The model under review builds one solid part; all positions refer to its coordinate system, in mm. A direction names the side the tool comes from. Round coordinates to 2 decimals unless told otherwise and drop trailing zeros. Order: outer loops, then holes, each group sorted by start corner. A loop starts at its lowest first (then second) coordinate and runs counter-clockwise, first axis right, second up. Notation, with made-up numbers: M 49.5,63 L 94.5,63 A27 cw 94.5,85 Z; hole C 71.25,-18 d3. An arc over 180 degrees is marked long. Answer as a JSON object with one key per item and string values. Group by question number.
1. Add section A-A on z = -5.5. State the section outline as (x, y) points.
2. To check wall thickness, follow probe 1 along Z at (x, y) = (-7, 4.5); probe 2 along Z at (x, y) = (5.5, 2); probe 3 along Y at (x, z) = (-18.5, -4). State the ranges of each line that lie inside material, in increasing order. Write a range as [from, to].
3. Add section B-B on y = 6.5. State the section outline as (x, z) points, and give its area (3 significant figures).
4. Add section D-D on z = -2. State the section outline as (x, y) points.
5. Add section C-C on x = 9. State the section outline as (y, z) points, and give its area (3 significant figures).
6. Machinability: for faces 4 (the face through (0.2, 7, -13.2)), 5 (the face through (-24, 5, 12)), 6 (the face through (0, 3, -14)), 7 (the face through (-25.507, 4.65, 3.736)), 8 (the face through (-22.855, 1.15, -11.43)), which of the approach directions +Z, -Z, +X, -X, +Y, -Y give a long, thin tool a straight path to every point of the face, cutting with its end or side? Answer none if there is none.
7. Mouldability with a two-part tool opening along X and no side actions: class faces 1 (the face through (0, 5, -13)), 2 (the face through (23.5, 3, 12)), 3 (the face through (0, 0, 0)) as released by +X, released by -X, zero draft, split by the parting line, or undercut.
8. Clearance check with flat-ended pins moving along their axes: P1, Ø5, axis at x = -6.5, z = 4, coming from the +Y side; P2, Ø1.6, axis at x = -22.5, z = -12, coming from the +Y side; P3, Ø0.6, axis at x = -25, y = 6.5, coming from the -Z side. State where each tip first meets the part, or that it passes through.
```python
from build123d import *

# Parameters (mm, degrees)
SKETCH_1_W          = 52
SKETCH_1_H          = 28
EXTRUDE_1_DEPTH     = 6
SKETCH_3_W          = 51
SKETCH_3_H          = 26
CUT_EXTRUDE_1_DEPTH = 5
SKETCH_4_W          = 10
SKETCH_4_H          = 1
EXTRUDE_2_DEPTH     = 4
CUT_EXTRUDE_2_REACH = 56.185
FILLET_1_R          = 0.5
EXTRUDE_3_DEPTH     = 1
CHAMFER_1_SIZE      = 0.1
CHAMFER_1_SIZE_2    = 1


# Some blends are built 0.0001 mm under size
with BuildPart() as part:
    # Эскиз1 → Бобышка-Вытянуть1 (new body)
    with BuildSketch(Plane(origin=(0, 0, 0), x_dir=(1, 0, 0), z_dir=(0, 1, 0))):
        Rectangle(SKETCH_1_W, SKETCH_1_H)
    extrude(amount=EXTRUDE_1_DEPTH)

    # Эскиз3 → Вырез-Вытянуть1 (cut)
    with BuildSketch(Plane(origin=(0, 6, 0), x_dir=(1, 0, 0), z_dir=(0, 1, 0))):
        with Locations((0.5, 0)):
            Rectangle(SKETCH_3_W, SKETCH_3_H)
    extrude(amount=-CUT_EXTRUDE_1_DEPTH, mode=Mode.SUBTRACT)

    # Эскиз4 → Бобышка-Вытянуть2 (add)
    with BuildSketch(Plane(origin=(0, 1, 0), x_dir=(1, 0, 0), z_dir=(0, 1, 0))):
        Polygon((19.5, 13), (23.5, 10), (23.5, 13), align=None)
        Polygon((-25, 13), (-25, 10), (-21, 13), align=None)
        Polygon((-21, -13), (-25, -13), (-25, -10), align=None)
        Polygon((23.5, -13), (19.5, -13), (23.5, -10), align=None)
        with Locations((-10, 0)):
            Rectangle(SKETCH_4_W, SKETCH_4_H)
    extrude(amount=EXTRUDE_2_DEPTH)

    # Эскиз5 → Вырез-Вытянуть2 (cut, up to next)
    with BuildSketch(Plane.ZY.offset(26), mode=Mode.PRIVATE) as cut_extrude_2_sk1:
        with BuildLine():
            Line((2.5, 4), (-2.5, 4))
            ThreePointArc((-2.5, 4), (-4, 5.5), (-2.5, 7))
            Line((-2.5, 7), (2.5, 7))
            ThreePointArc((2.5, 7), (4, 5.5), (2.5, 4))
        make_face()
    cut_extrude_2_tool1 = extrude(cut_extrude_2_sk1.sketch, amount=-CUT_EXTRUDE_2_REACH, mode=Mode.PRIVATE) & part.part
    add(cut_extrude_2_tool1.solids().sort_by_distance((-26, 5.5, 0))[0], mode=Mode.SUBTRACT)

    # Скругление1
    fillet_1_edges = [part.edges().sort_by_distance(p)[0] for p in [
        (-26, 3, -14),
        (26, 3, -14),
        (0, 0, -14),
        (-26, 0, 0),
        (-26, 3, 14),
        (26, 0, 0),
        (26, 3, 14),
        (0, 0, 14),
        (-21, 3, 13),
        (-0.75, 1, 13),
        (19.5, 3, 13),
        (-23, 1, -11.5),
        (-25, 1, 0),
        (-23, 1, 11.5),
        (21.5, 1, 11.5),
        (23.5, 1, 11.5),
        (23.5, 1, -11.5),
        (21.5, 1, -11.5),
        (-0.75, 1, -13),
        (-10, 1, -0.5),
        (-5, 1, 0),
        (-10, 1, 0.5),
        (-15, 1, 0),
        (19.5, 3, -13),
        (-21, 3, -13),
        (-25, 3, -10),
        (-25, 3, 10),
        (23.5, 3, 10),
        (23.5, 3, -10),
        (-15, 3, -0.5),
        (-5, 3, -0.5),
        (-10, 5, -0.5),
        (-5, 3, 0.5),
        (-15, 3, 0.5),
        (-10, 5, 0.5),
    ]]
    fillet(fillet_1_edges, radius=FILLET_1_R - 0.0001)  # a hair under: the kernel refuses the full size

    # Эскиз6 → Бобышка-Вытянуть3 (add)
    with BuildSketch(Plane(origin=(0, 6, 0), x_dir=(1, 0, 0), z_dir=(0, 1, 0))):
        Polygon((-25.5, 3.914213562), (-25, 3.914213562), (-25, 13), (26, 13), (26, 13.5), (-25.5, 13.5), align=None)
        Polygon((-25.5, -13.5), (-25.5, -3.914213562), (-25, -3.914213562), (-25, -13), (26, -13), (26, -13.5), align=None)
    extrude(amount=EXTRUDE_3_DEPTH)

    # Фаска1
    # the kernel refuses this chamfer: 1, 0.1 mm, written as the material it takes off along each edge
    with BuildSketch(Plane(origin=(28.599522763, 7, 13.5), x_dir=(0, 0.3574851447578448, -0.9339188247794681), z_dir=(-1, 0, 0))) as chamfer_1_piece_1_section:
        Polygon((CHAMFER_1_SIZE * 0.933918824779, CHAMFER_1_SIZE * 0.357485144758), (-CHAMFER_1_SIZE_2 * 0.357485144758, CHAMFER_1_SIZE_2 * 0.933918824779), (0, 0), align=None)
    chamfer_1_piece_1 = extrude(amount=56.699045526, mode=Mode.PRIVATE)
    chamfer_1_piece_1 = split(chamfer_1_piece_1, bisect_by=Plane(origin=(0.25, 6, 13.477938847), z_dir=(0, 1, 0)), keep=Keep.TOP, mode=Mode.PRIVATE)
    add(chamfer_1_piece_1, mode=Mode.SUBTRACT)
    with BuildSketch(Plane(origin=(-25.5, 7, 16.099522763), x_dir=(-0.003827768713514726, -0.9999926740665033, 0), z_dir=(0, 0, -1))) as chamfer_1_piece_2_section:
        Polygon((CHAMFER_1_SIZE_2 * 0.999992674067, -CHAMFER_1_SIZE_2 * 0.00382776871351), (-CHAMFER_1_SIZE * 0.00382776871351, -CHAMFER_1_SIZE * 0.999992674067), (0, 0), align=None)
    chamfer_1_piece_2 = extrude(amount=14.784831964, mode=Mode.PRIVATE)
    chamfer_1_piece_2 = split(chamfer_1_piece_2, bisect_by=Plane(origin=(-25.477938847, 6, 8.707106781), z_dir=(0, 1, 0)), keep=Keep.TOP, mode=Mode.PRIVATE)
    add(chamfer_1_piece_2, mode=Mode.SUBTRACT)
    with BuildSketch(Plane(origin=(28.599522763, 7, -13.5), x_dir=(0, 0.3574851447578448, 0.9339188247794681), z_dir=(-1, 0, 0))) as chamfer_1_piece_3_section:
        Polygon((CHAMFER_1_SIZE * 0.933918824779, -CHAMFER_1_SIZE * 0.357485144758), (-CHAMFER_1_SIZE_2 * 0.357485144758, -CHAMFER_1_SIZE_2 * 0.933918824779), (0, 0), align=None)
    chamfer_1_piece_3 = extrude(amount=56.699045526, mode=Mode.PRIVATE)
    chamfer_1_piece_3 = split(chamfer_1_piece_3, bisect_by=Plane(origin=(0.25, 6, -13.477938847), z_dir=(0, 1, 0)), keep=Keep.TOP, mode=Mode.PRIVATE)
    add(chamfer_1_piece_3, mode=Mode.SUBTRACT)
    with BuildSketch(Plane(origin=(-25.5, 7, -16.099522763), x_dir=(0.9339188247794681, 0.3574851447578448, 0), z_dir=(0, 0, 1))) as chamfer_1_piece_4_section:
        Polygon((CHAMFER_1_SIZE * 0.933918824779, -CHAMFER_1_SIZE * 0.357485144758), (-CHAMFER_1_SIZE_2 * 0.357485144758, -CHAMFER_1_SIZE_2 * 0.933918824779), (0, 0), align=None)
    chamfer_1_piece_4 = extrude(amount=14.784831964, mode=Mode.PRIVATE)
    chamfer_1_piece_4 = split(chamfer_1_piece_4, bisect_by=Plane(origin=(-25.477938847, 6, -8.707106781), z_dir=(0, 1, 0)), keep=Keep.TOP, mode=Mode.PRIVATE)
    add(chamfer_1_piece_4, mode=Mode.SUBTRACT)


solid = part.part
```
Recorded:
{
 "1": {"outline": "M -26,0.5 A0.5 ccw -25.5,0 L 25.5,0 A0.5 ccw 26,0.5 L 26,1 L -24.5,1 A0.5 cw -25,1.5 L -25,7 L -25.4,7 L -25.5,6 L -26,6 Z"},
 "2": {"probe 1": "z = [-14, -13], [-0.5, 0.5], [13, 14]", "probe 2": "z = [-14, -13], [13, 14]", "probe 3": "y = [0, 1]"},
 "3": {"outline": "M -25.45,-13.45 L 26,-13.45 L 26,-13 L -25,-13 L -25,-3.91 L -25.45,-3.91 Z; M -25.45,3.91 L -25,3.91 L -25,13 L 26,13 L 26,13.45 L -25.45,13.45 Z", "area": "54.5 mm²"},
 "4": {"outline": "M -26,0.5 A0.5 ccw -25.5,0 L 25.5,0 A0.5 ccw 26,0.5 L 26,1 L -24.5,1 A0.5 cw -25,1.5 L -25,4 L -26,4 Z"},
 "5": {"outline": "M 0,-13.5 A0.5 ccw 0.5,-14 L 6,-14 L 6,-13.5 L 7,-13.4 L 7,-13 L 1.5,-13 A0.5 cw 1,-12.5 L 1,12.5 A0.5 cw 1.5,13 L 7,13 L 7,13.4 L 6,13.5 L 6,14 L 0.5,14 A0.5 ccw 0,13.5 Z", "area": "38.9 mm²"},
 "6": {"face 4": "+Z, -Z, +X, -X, +Y", "face 5": "+X, +Y", "face 6": "-Z, +X, -X, +Y, -Y", "face 7": "+X, -X", "face 8": "+Y"},
 "7": {"face 1": "undercut", "face 2": "released by +X", "face 3": "zero draft"},
 "8": {"P1": "stops at y = 1", "P2": "stops at y = 5", "P3": "stops at z = -13.48"}
}
